from build123d import *

# Parameters (mm, degrees)
SALIENTE_EXTRUIR1_DEPTH = 3
SALIENTE_EXTRUIR2_DEPTH = 17.5
REDONDEO1_R             = 3.175
REDONDEO3_R             = 3.175
REDONDEO5_R             = 3.175
CROQUIS5_R              = 1.5
CORTAR_EXTRUIR1_DEPTH   = 10
SALIENTE_EXTRUIR3_DEPTH = 7
REDONDEO6_R             = 3.175
REDONDEO7_R             = 3.175
REDONDEO8_R             = 3.175
REDONDEO12_R            = 20
REDONDEO11_R            = 20


with BuildPart() as part:
    # Croquis2 → Saliente-Extruir1 (new body)
    with BuildSketch(Plane(origin=(0, 0, 0), x_dir=(1, 0, 0), z_dir=(0, 1, 0))):
        with BuildLine():
            Line((-98.5, -27.5), (-98.5, -66.771770067))
            Line((-98.5, -66.771770067), (0, -84.139977667))
            Line((0, -84.139977667), (98.5, -66.771770067))
            Line((98.5, -66.771770067), (98.5, -27.5))
            Line((98.5, -27.5), (79.5, -27.5))
            Line((79.5, -27.5), (79.5, -19))
            Line((79.5, -19), (59.5, -19))
            Line((59.5, -19), (59.5, 19))
            Line((59.5, 19), (79.5, 19))
            Line((79.5, 19), (79.5, 27.5))
            Line((79.5, 27.5), (98.5, 27.5))
            Line((98.5, 27.5), (98.5, 36.239787367))
            Line((98.5, 36.239787367), (79.5, 39.59))
            Line((79.5, 39.59), (33.578271315, 39.59))
            Line((33.578271315, 39.59), (29.885840943, -2.614672282))
            ThreePointArc((29.885840943, -2.614672282), (0, -30), (-29.885840943, -2.614672282))
            Line((-29.885840943, -2.614672282), (-33.578271315, 39.59))
            Line((-33.578271315, 39.59), (-79.5, 39.59))
            Line((-79.5, 39.59), (-98.5, 36.239787367))
            Line((-98.5, 36.239787367), (-98.5, 27.5))
            Line((-98.5, 27.5), (-79.5, 27.5))
            Line((-79.5, 27.5), (-79.5, 19))
            Line((-79.5, 19), (-54.5, 19))
            Line((-54.5, 19), (-54.5, -19))
            Line((-54.5, -19), (-79.5, -19))
            Line((-79.5, -19), (-79.5, -27.5))
            Line((-79.5, -27.5), (-98.5, -27.5))
        make_face()
    extrude(amount=SALIENTE_EXTRUIR1_DEPTH)

    # Croquis2<3> → Saliente-Extruir2 (add)
    with BuildSketch(Plane(origin=(0, 0, 0), x_dir=(1, 0, 0), z_dir=(0, 1, 0))):
        with BuildLine():
            Line((-98.5, -27.5), (-98.5, -66.771770067))
            Line((-98.5, -66.771770067), (0, -84.139977667))
            Line((0, -84.139977667), (98.5, -66.771770067))
            Line((98.5, -66.771770067), (98.5, -27.5))
            Line((98.5, -27.5), (79.5, -27.5))
            Line((79.5, -27.5), (79.5, -19))
            Line((79.5, -19), (59.5, -19))
            Line((59.5, -19), (59.5, -10))
            Line((59.5, -10), (35, -10))
            Line((35, -10), (35, 10))
            Line((35, 10), (59.5, 10))
            Line((59.5, 10), (59.5, 19))
            Line((59.5, 19), (79.5, 19))
            Line((79.5, 19), (79.5, 27.5))
            Line((79.5, 27.5), (98.5, 27.5))
            Line((98.5, 27.5), (98.5, 36.239787367))
            Line((98.5, 36.239787367), (79.5, 39.59))
            Line((79.5, 39.59), (33.578271315, 39.59))
            Line((33.578271315, 39.59), (29.885840943, -2.614672282))
            ThreePointArc((29.885840943, -2.614672282), (0, -30), (-29.885840943, -2.614672282))
            Line((-29.885840943, -2.614672282), (-33.578271315, 39.59))
            Line((-33.578271315, 39.59), (-79.5, 39.59))
            Line((-79.5, 39.59), (-98.5, 36.239787367))
            Line((-98.5, 36.239787367), (-98.5, 27.5))
            Line((-98.5, 27.5), (-79.5, 27.5))
            Line((-79.5, 27.5), (-79.5, 19))
            Line((-79.5, 19), (-54.5, 19))
            Line((-54.5, 19), (-54.5, 10))
            Line((-54.5, 10), (-35, 10))
            Line((-35, 10), (-35, -10))
            Line((-35, -10), (-54.5, -10))
            Line((-54.5, -10), (-54.5, -19))
            Line((-54.5, -19), (-79.5, -19))
            Line((-79.5, -19), (-79.5, -27.5))
            Line((-79.5, -27.5), (-98.5, -27.5))
        make_face()
        Polygon((-36.327264837, 36.59), (-34.263407265, 13), (-51.5, 13), (-51.5, 22), (-71.5, 22), (-71.5, 30.5), (-93.5, 30.5), (-93.5, 34.12142227), (-79.5, 36.59), align=None, mode=Mode.SUBTRACT)
        with BuildLine():
            Line((0, -76.016564772), (-93.5, -59.529992076))
            Line((-93.5, -59.529992076), (-93.5, -30))
            Line((-93.5, -30), (-71.5, -30))
            Line((-71.5, -30), (-71.5, -24))
            Line((-71.5, -24), (-49.5, -24))
            Line((-49.5, -24), (-49.5, -15))
            Line((-49.5, -15), (-29.393876913, -15))
            ThreePointArc((-29.393876913, -15), (0, -33), (29.393876913, -15))
            Line((29.393876913, -15), (49.5, -15))
            Line((49.5, -15), (49.5, -24))
            Line((49.5, -24), (71.5, -24))
            Line((71.5, -24), (71.5, -30))
            Line((71.5, -30), (93.5, -30))
            Line((93.5, -30), (93.5, -59.529992076))
            Line((93.5, -59.529992076), (0, -76.016564772))
        make_face(mode=Mode.SUBTRACT)
        Polygon((71.5, 30.5), (71.5, 22), (51.5, 22), (51.5, 13), (34.263407265, 13), (36.327264837, 36.59), (79.5, 36.59), (93.5, 34.12142227), (93.5, 30.5), align=None, mode=Mode.SUBTRACT)
    extrude(amount=SALIENTE_EXTRUIR2_DEPTH)

    # Redondeo1
    # the kernel refuses this fillet: 3.175 mm, written as the material it adds along each edge
    with BuildSketch(Plane(origin=(-79.5, 2.305558733, -36.59), x_dir=(1, 0, 0), z_dir=(0, 1, 0))) as redondeo1_piece_1:
        with BuildLine():
            CenterArc((REDONDEO1_R * 0.0874886635259, -REDONDEO1_R), REDONDEO1_R, 90, 10)
            Line((-REDONDEO1_R * 0.086159514141, -REDONDEO1_R * 0.0151922469878), (0, 0))
            Line((0, 0), (REDONDEO1_R * 0.0874886635259, 0))
        make_face()
    extrude(amount=15.194441267)
    with BuildSketch(Plane(origin=(-51.5, 3, -13), x_dir=(0, 0, -1), z_dir=(0, 1, 0)), Plane(origin=(-71.5, 3, -22), x_dir=(0, 0, -1), z_dir=(0, 1, 0)), Plane(origin=(-93.5, 3, -30.5), x_dir=(0, 0, -1), z_dir=(0, 1, 0))) as redondeo1_piece_2:
        with BuildLine():
            CenterArc((REDONDEO1_R, -REDONDEO1_R), REDONDEO1_R, 90, 90)
            Line((0, -REDONDEO1_R), (0, 0))
            Line((0, 0), (REDONDEO1_R, 0))
        make_face()
    extrude(amount=14.5)
    with BuildSketch(Plane(origin=(-93.5, 3, -34.12142227), x_dir=(0.9848077530122092, 0, -0.17364817766692342), z_dir=(0, 1, 0))) as redondeo1_piece_3:
        with BuildLine():
            CenterArc((REDONDEO1_R * 0.839099631177, -REDONDEO1_R), REDONDEO1_R, 90, 80)
            Line((-REDONDEO1_R * 0.145708121835, -REDONDEO1_R * 0.826351822333), (0, 0))
            Line((0, 0), (REDONDEO1_R * 0.839099631177, 0))
        make_face()
    extrude(amount=14.5)

    # Redondeo3
    redondeo3_edges = [part.edges().sort_by_distance(p)[0] for p in [
        (-49.5, 10.25, 15),
        (-29.393876913, 10.25, 15),
        (29.393876913, 10.25, 15),
        (49.5, 10.25, 15),
        (71.5, 10.25, 24),
        (93.5, 10.25, 30),
        (93.5, 10.25, 59.529992076),
        (0, 10.25, 76.016564772),
        (-93.5, 10.25, 59.529992076),
        (-93.5, 10.25, 30),
        (-71.5, 10.25, 24),
    ]]
    fillet(redondeo3_edges, radius=REDONDEO3_R)

    # Redondeo5
    redondeo5_edges = [part.edges().sort_by_distance(p)[0] for p in [
        (-49.5, 10.25, 24),
        (-71.5, 10.25, 30),
        (71.5, 10.25, 30),
        (49.5, 10.25, 24),
        (71.5, 10.25, -30.5),
        (51.5, 10.25, -22),
        (-51.5, 10.25, -22),
        (-71.5, 10.25, -30.5),
    ]]
    fillet(redondeo5_edges, radius=REDONDEO5_R)

    # Croquis5 → Cortar-Extruir1 (cut)
    with BuildSketch(Plane(origin=(0, 17.5, 0), x_dir=(1, 0, 0), z_dir=(0, 1, 0))):
        with Locations(Location((0, -80.053781473, 0), (0, 0, 270))):
            Circle(CROQUIS5_R)
        with Locations(Location((-94.5, -63.390881796, 0), (0, 0, 270))):
            Circle(CROQUIS5_R)
        with Locations(Location((-75.5, -23.25, 0), (0, 0, 270))):
            Circle(CROQUIS5_R)
        with Locations(Location((-75.5, 23.25, 0), (0, 0, 90))):
            Circle(CROQUIS5_R)
        with Locations(Location((75.5, 23.25, 0), (0, 0, 270))):
            Circle(CROQUIS5_R)
        with Locations(Location((95.718468624, 31.869893683, 0), (0, 0, 90))):
            Circle(CROQUIS5_R)
        with Locations(Location((75.5, -23.25, 0), (0, 0, 90))):
            Circle(CROQUIS5_R)
        with Locations(Location((94.5, -63.390881796, 0), (0, 0, 90))):
            Circle(CROQUIS5_R)
    extrude(amount=-CORTAR_EXTRUIR1_DEPTH, mode=Mode.SUBTRACT)

    # Croquis2<4> → Saliente-Extruir3 (add)
    with BuildSketch(Plane(origin=(0, 0, 0), x_dir=(1, 0, 0), z_dir=(0, 1, 0))):
        Polygon((-54.5, 10), (-54.5, -10), (-37.5, -10), (-35, -10), (-35, 10), (-37.5, 10), align=None)
        Polygon((37.5, -10), (59.5, -10), (59.5, 10), (37.5, 10), (35, 10), (35, -10), align=None)
    extrude(amount=SALIENTE_EXTRUIR3_DEPTH)

    # Redondeo6
    redondeo6_edges = [part.edges().sort_by_distance(p)[0] for p in [
        (-35, 12.25, -10),
        (-35, 12.25, 10),
        (35, 12.25, 10),
        (35, 12.25, -10),
        (79.5, 8.75, -27.5),
        (59.5, 8.75, -19),
        (59.5, 8.75, 19),
        (79.5, 8.75, 27.5),
        (-79.5, 8.75, 27.5),
        (-54.5, 8.75, 19),
        (-54.5, 8.75, -19),
        (-79.5, 8.75, -27.5),
    ]]
    fillet(redondeo6_edges, radius=REDONDEO6_R)

    # Redondeo7
    redondeo7_edges = [part.edges().sort_by_distance(p)[0] for p in [
        (-34.263407265, 10.25, -13),
    ]]
    fillet(redondeo7_edges, radius=REDONDEO7_R)

    # Redondeo8
    redondeo8_edges = [part.edges().sort_by_distance(p)[0] for p in [
        (34.263407265, 10.25, -13),
        (79.5, 10.25, -36.59),
        (71.5, 10.25, -22),
        (51.5, 10.25, -13),
    ]]
    fillet(redondeo8_edges, radius=REDONDEO8_R)

    # Redondeo12
    redondeo12_edges = [part.edges().sort_by_distance(p)[0] for p in [
        (36.327264837, 10.25, -36.59),
        (-36.327264837, 10.25, -36.59),
    ]]
    fillet(redondeo12_edges, radius=REDONDEO12_R)

    # Redondeo11
    redondeo11_edges = [part.edges().sort_by_distance(p)[0] for p in [
        (-33.578271315, 8.75, -39.59),
        (33.578271315, 8.75, -39.59),
    ]]
    fillet(redondeo11_edges, radius=REDONDEO11_R)


solid = part.part
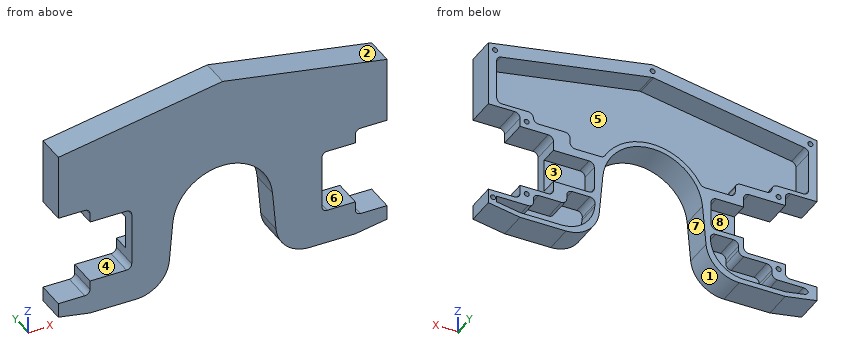
For this review, take the finished solid that the model builds, in its own axes (mm). Face numbers are marked on the shaded views. A direction names the side the tool comes from. Give positions to 0.01 mm unless a question says otherwise; leave off trailing zeros. Loops run counter-clockwise (first coordinate to the right, second up) from the corner with the lowest first, then second, coordinate; pieces in that order, holes last. Notation, with made-up numbers: M -25.5,-2 L 10.5,-2 A7 ccw 10.5,10 Z; hole C 74.5,53 d10. An arc over 180 degrees is marked long. Put each result on its own line as item: value. Start each with the question number.
(1) For pin 1 (12 mm diameter, centred on x = 58.5, z = -5, fed in from +Y); pin 2 (8.5 mm diameter, centred on x = 47, y = 11, fed in from +Z); pin 3 (7 mm diameter, centred on x = 84.5, y = 8.5, fed in from -Z); pin 4 (1.3 mm diameter, centred on y = 11, z = -17.5, fed in from -X), all flat-tipped, find the tip position at first contact; note any pin that passes through.
(2) Machinability: for the marked faces 4, 5, 6, 7 and 8, which of the approach directions +Z, -Z, +X, -X, +Y, -Y give a long, thin tool a straight path to every point of the face, cutting with its end or side? Answer none if there is none.
(3) Add section C-C, the plane y = 10.5. Give the number of separate pieces and of enclosed holes in the cut face, then the cut area to 3 significant figures.
(4) The part is to be moulded in two halves that separate along X. For the marked faces 1, 2 and 3, say which applies: +X half, -X half, draft (parallel to the pull), parting line (faces both ways), or undercut.
(5) Add section A-A, the plane z = 50.5. Write out the cut boundary in (x, y), then the cut area to 3 significant figures.
(6) Wall thickness on L1, parallel to X at y = 13.75, z = 33.5; L2, parallel to X at y = 16.5, z = -24; L3, parallel to Z at x = -94.5, y = 14.5: over which ranges is each line inside the solid? List them lowest first.
(7) Add section B-B, the plane x = -16. Write out the cut boundary in (y, z).
Result:
1. pin 1: stops at y = 17.5
1. pin 2: stops at z = 76.6
1. pin 3: stops at z = -39.33
1. pin 4: stops at x = -55.51
2. face 4: -X, +Y, -Y
2. face 5: +Y
2. face 6: +X, +Y, -Y
2. face 7: -Z, +Y, -Y
2. face 8: -X, +Y
3. separate pieces: 1
3. enclosed holes: 11
3. area: 4,330 mm^2
4. face 1: undercut
4. face 2: +X half
4. face 3: draft
5. outline: M -98.5,0 L 98.5,0 L 98.5,17.5 L 93.5,17.5 L 93.5,3 L -93.5,3 L -93.5,17.5 L -98.5,17.5 Z
5. area: 736 mm^2
6. L1: x = -98.5 to -93.5, 93.5 to 98.5
6. L2: x = -79.5 to -76.8, -74.2 to -71.27, -36.08 to -32.4, 32.4 to 36.08, 71.27 to 74.2, 76.8 to 79.5
6. L3: z = -36.95 to -27.5, 27.5 to 61.89, 64.89 to 67.48
7. outline: M 0,25.38 L 17.5,25.38 L 17.5,28.86 L 3,28.86 L 3,73.2 L 17.5,73.2 L 17.5,81.32 L 0,81.32 Z
